Part model, mm, in its own coordinate system. Give positions to 0.01 mm unless a question says otherwise; leave off trailing zeros. Order: outer loops, then holes, each group sorted by start corner. A loop starts at its lowest first (then second) coordinate and runs counter-clockwise, first axis right, second up.
1. Slice it at A-A on z = 9. List the corners of the cut face in (x, y).
2. Drop flat-ended pins along their axis: pin 1 Ø8 at (x, z) = (17, 6.5) entering from -Y; pin 2 Ø14.5 at (y, z) = (-30.5, 20) entering from +X; pin 3 Ø8 at (y, z) = (-426.5, 25.5) entering from +X (3 decimals). Give the stop position or say it passes through.
3. Slice it at C-C on x = 397.5. List the corners of the cut face in (y, z) (1 decimal), and give its area (3 significant figures).
4. Slice it at B-B on y = -46.5. List the corners of the cut face in (x, z) (3 decimals).
5. Probe line 1 (X direction, y = -44.5, z = 26.5); line 2 (X direction, y = 142.5, z = 4); line 3 (Y direction, x = -381.5, z = 24.5). List the from-to ranges inside material, lowest first.
6. Slice it at D-D on y = 157.5. List the corners of the cut face in (x, z) (3 decimals), and give its area (3 significant figures).
from build123d import *

# Parameters (mm, degrees)
F0_W     = 127
F0_H     = 101.6
F1_DEPTH = 28.575


with BuildPart() as f1:
    # F0 (on Top) → F1 (new body)
    with BuildSketch(Plane.XY):
        Polygon((298.114391, -805.786025), (571.5, 0), (361.614391, 0), (361.614391, -101.6), (298.114391, -101.6), align=None)
        Polygon((298.114391, 101.6), (298.114391, 805.786025), (-444.5, 635), (-444.5, 0), (-63.5, 0), (-63.5, 101.6), (63.5, 101.6), (63.5, 0), (234.614391, 0), (234.614391, 101.6), align=None)
        Polygon((361.614391, 0), (571.5, 0), (298.114391, 805.786025), (298.114391, 101.6), (361.614391, 101.6), align=None)
        Polygon((-444.5, -635), (298.114391, -805.786025), (298.114391, -101.6), (234.614391, -101.6), (234.614391, 0), (63.5, 0), (63.5, -101.6), (-63.5, -101.6), (-63.5, 0), (-444.5, 0), align=None)
        with Locations((0, 50.8)):
            Rectangle(F0_W, F0_H)
        with Locations((0, -50.8)):
            Rectangle(F0_W, F0_H)
    extrude(amount=F1_DEPTH)


solid = f1.part
Data:
1. outline: (-444.5, -635) - (298.11, -805.79) - (571.5, 0) - (298.11, 805.79) - (-444.5, 635) - close; hole (234.61, -101.6) - (361.61, -101.6) - (361.61, 101.6) - (234.61, 101.6) - close
2. pin 1: stops at y = -742.06
2. pin 2: stops at x = 563.61
2. pin 3: stops at x = 428.155
3. outline: (-512.9, 0) - (512.9, 0) - (512.9, 28.6) - (-512.9, 28.6) - close
3. area: 29,300 mm2
4. outline: (-444.5, 0) - (234.614, 0) - (234.614, 28.575) - (-444.5, 28.575) - close; (361.614, 0) - (555.724, 0) - (555.724, 28.575) - (361.614, 28.575) - close
5. line 1: x = -444.5 to 234.61, 361.61 to 556.4
5. line 2: x = -444.5 to 523.15
5. line 3: y = -649.49 to 649.49
6. outline: (-444.5, 0) - (518.064, 0) - (518.064, 28.575) - (-444.5, 28.575) - close
6. area: 27,500 mm2
